Part print with two shaded views. Sizes in mm from the minimum x, y, z corner. Round coordinates to 2 decimals unless told otherwise and drop trailing zeros. Loops run counter-clockwise (first coordinate to the right, second up) from the corner with the lowest first, then second, coordinate; pieces in that order, holes last. Notation, with made-up numbers: M 29,36.25 L 60,36.25 A14 ccw 60,47.25 Z; hole C 68,-10.75 d6. An arc over 180 degrees is marked long. Use a Markdown table: item, result. Add a question column.
Item 1: Saw through at C-C on z = 38. Write the cut outline in (x, y), then the cut area to 3 significant figures.
Item 2: Saw through at B-B on y = 2.2. Write the cut outline in (x, z), then the cut area to 3 significant figures.
Item 3: Wall check: L1, parallel to X at y = 1, z = 38; L2, parallel to X at y = 4.5, z = 70; L3, parallel to Z at x = 10.5, y = 3.45. Give the ranges that are in metal, low to high. Write a range as from..to.
Item 4: Pin check, flat tips, straight feed: P1, Ø2.5, axis at y = 2.5, z = 2.5, coming from the +X side; P2, Ø1.5, axis at x = 65, y = 2.5, coming from the -Z side; P3, Ø2.5, axis at y = 3.5, z = 70.5, coming from the -X side. Stop position of each tip, or through.
Item 5: Saw through at A-A on x = 37.5. Write the cut outline in (y, z).
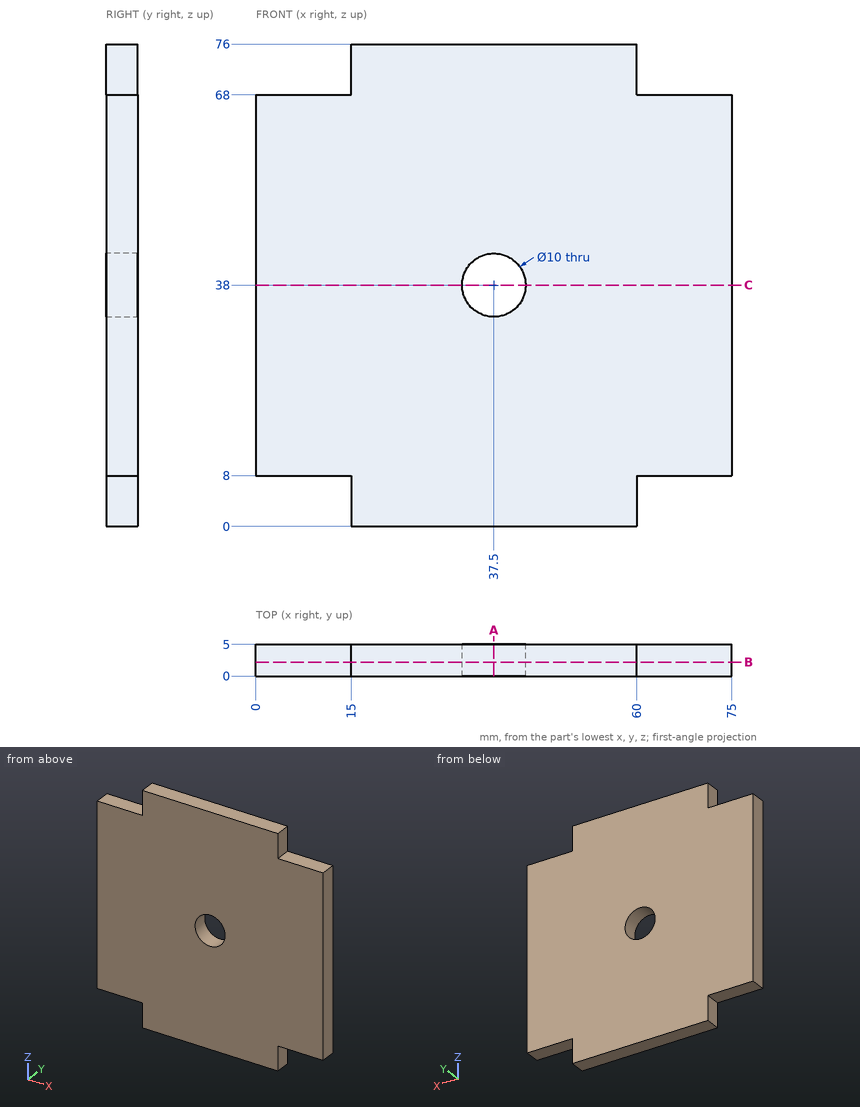
Entries:
| question | item | result |
|---|---|---|
| 1 | outline | M 0,0 L 32.5,0 L 32.5,5 L 0,5 Z; M 42.5,0 L 75,0 L 75,5 L 42.5,5 Z |
| 1 | area | 325 mm2 |
| 2 | outline | M 0,8 L 15,8 L 15,0 L 60,0 L 60,8 L 75,8 L 75,68 L 60,68 L 60,76 L 15,76 L 15,68 L 0,68 Z; hole C 37.5,38 d10 |
| 2 | area | 5,140 mm2 |
| 3 | L1 | 0..32.5, 42.5..75 |
| 3 | L2 | 15..60 |
| 3 | L3 | 8..68 |
| 4 | P1 | x = 60 |
| 4 | P2 | z = 8 |
| 4 | P3 | x = 15 |
| 5 | outline | M 0,0 L 5,0 L 5,33 L 0,33 Z; M 0,43 L 5,43 L 5,76 L 0,76 Z |
